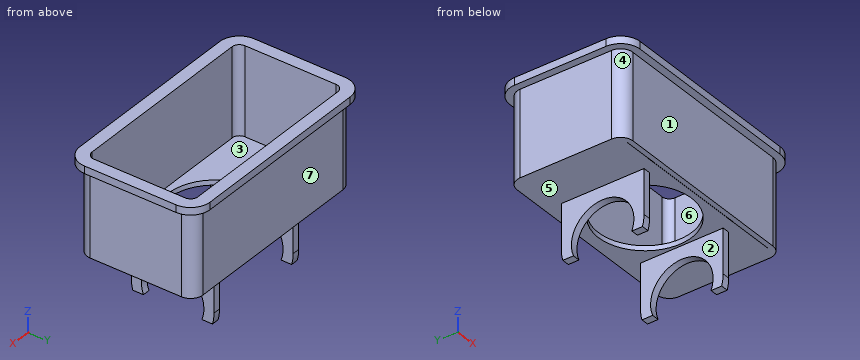
from build123d import *

# Parameters (mm, degrees)
BOSS_EXTRUDE1_DEPTH = 3
BOSS_EXTRUDE2_START = -38
BOSS_EXTRUDE2_DEPTH = 38
SKETCH3_R           = 19
BOSS_EXTRUDE3_DEPTH = 2
SKETCH4_W           = 3
SKETCH4_H           = 42
BOSS_EXTRUDE4_DEPTH = 35
CUT_EXTRUDE1_START  = -46
SKETCH5_R           = 12.75
CUT_EXTRUDE1_DEPTH  = 46
CUT_EXTRUDE2_REACH  = 103.826
CUT_EXTRUDE3_REACH  = 103.826
SKETCH7_W           = 14.582252834
SKETCH7_H           = 33.756


with BuildPart() as part:
    # Sketch1 → Boss-Extrude1 (new body)
    with BuildSketch(Plane.XY):
        with BuildLine():
            Line((-38, 26.6), (38, 26.6))
            ThreePointArc((38, 26.6), (43.656854249, 24.256854249), (46, 18.6))
            Line((46, 18.6), (46, -18.6))
            ThreePointArc((46, -18.6), (43.656854249, -24.256854249), (38, -26.6))
            Line((38, -26.6), (-38, -26.6))
            ThreePointArc((-38, -26.6), (-43.656854249, -24.256854249), (-46, -18.6))
            Line((-46, -18.6), (-46, 18.6))
            ThreePointArc((-46, 18.6), (-43.656854249, 24.256854249), (-38, 26.6))
        make_face()
        with BuildLine():
            Line((-38, -23.6), (38, -23.6))
            ThreePointArc((38, -23.6), (41.535533906, -22.135533906), (43, -18.6))
            Line((43, -18.6), (43, 18.6))
            ThreePointArc((43, 18.6), (41.535533906, 22.135533906), (38, 23.6))
            Line((38, 23.6), (-38, 23.6))
            ThreePointArc((-38, 23.6), (-41.535533906, 22.135533906), (-43, 18.6))
            Line((-43, 18.6), (-43, -18.6))
            ThreePointArc((-43, -18.6), (-41.535533906, -22.135533906), (-38, -23.6))
        make_face(mode=Mode.SUBTRACT)
    extrude(amount=BOSS_EXTRUDE1_DEPTH)

    # Sketch2 → Boss-Extrude2 (add)
    with BuildSketch(Plane.XY.offset(3).offset(BOSS_EXTRUDE2_START)):
        with BuildLine():
            Line((43, 18.6), (43, -18.6))
            ThreePointArc((43, -18.6), (41.535533906, -22.135533906), (38, -23.6))
            Line((38, -23.6), (-38, -23.6))
            ThreePointArc((-38, -23.6), (-41.535533906, -22.135533906), (-43, -18.6))
            Line((-43, -18.6), (-43, 18.6))
            ThreePointArc((-43, 18.6), (-41.535533906, 22.135533906), (-38, 23.6))
            Line((-38, 23.6), (38, 23.6))
            ThreePointArc((38, 23.6), (41.535533906, 22.135533906), (43, 18.6))
        make_face()
        with BuildLine():
            ThreePointArc((41, 18.6), (40.121320344, 20.721320344), (38, 21.6))
            Line((38, 21.6), (-38, 21.6))
            ThreePointArc((-38, 21.6), (-40.121320344, 20.721320344), (-41, 18.6))
            Line((-41, 18.6), (-41, -18.6))
            ThreePointArc((-41, -18.6), (-40.121320344, -20.721320344), (-38, -21.6))
            Line((-38, -21.6), (38, -21.6))
            ThreePointArc((38, -21.6), (40.121320344, -20.721320344), (41, -18.6))
            Line((41, -18.6), (41, 18.6))
        make_face(mode=Mode.SUBTRACT)
    extrude(amount=BOSS_EXTRUDE2_DEPTH)

    # Sketch3 → Boss-Extrude3 (add)
    with BuildSketch(Plane(origin=(0, 0, -35), x_dir=(-1, 0, 0), z_dir=(0, 0, -1))):
        with BuildLine():
            ThreePointArc((41, 18.6), (40.121320344, 20.721320344), (38, 21.6))
            Line((38, 21.6), (-38, 21.6))
            ThreePointArc((-38, 21.6), (-40.121320344, 20.721320344), (-41, 18.6))
            Line((-41, 18.6), (-41, -18.6))
            ThreePointArc((-41, -18.6), (-40.365961681, -20.444512219), (-38.731849783, -21.509363486))
            Line((-38.731849783, -21.509363486), (38.731849783, -21.509363486))
            ThreePointArc((38.731849783, -21.509363486), (40.365961681, -20.444512219), (41, -18.6))
            Line((41, -18.6), (41, 18.6))
        make_face()
        Circle(SKETCH3_R, mode=Mode.SUBTRACT)
    extrude(amount=-BOSS_EXTRUDE3_DEPTH)

    # Sketch4 → Boss-Extrude4 (add)
    with BuildSketch(Plane(origin=(0, 0, -35), x_dir=(-1, 0, 0), z_dir=(0, 0, -1))):
        with Locations((-21.5, 2.6)):
            Rectangle(SKETCH4_W, SKETCH4_H)
        with Locations((21.5, 2.6)):
            Rectangle(SKETCH4_W, SKETCH4_H)
    extrude(amount=BOSS_EXTRUDE4_DEPTH)

    # Sketch5 → Cut-Extrude1 (cut)
    with BuildSketch(Plane.ZY.offset(23).offset(CUT_EXTRUDE1_START)):
        with Locations(Location((-53.122, 0, 0), (0, 0, 270))):
            Circle(SKETCH5_R)
    extrude(amount=CUT_EXTRUDE1_DEPTH, mode=Mode.SUBTRACT)

    # Cut-Extrude2: up to this face of the body (flat: up to its plane)
    cut_extrude2_end = Plane(part.part.faces().sort_by_distance((23, -17.853282523, -52.5))[0])
    # Sketch6 → Cut-Extrude2 (cut, up to the picked face)
    with BuildSketch(Plane.ZY.offset(23), mode=Mode.PRIVATE) as cut_extrude2_sk1:
        with BuildLine():
            ThreePointArc((-53.122, -16.878), (-65.056548253, -11.934548253), (-70, 0))
            Line((-70, 0), (-70, -18.4))
            Line((-70, -18.4), (-35, -18.4))
            Line((-35, -18.4), (-35, -16.878))
            Line((-35, -16.878), (-53.122, -16.878))
        make_face()
    cut_extrude2_tool1 = split(extrude(cut_extrude2_sk1.sketch, amount=-CUT_EXTRUDE2_REACH, mode=Mode.PRIVATE), bisect_by=cut_extrude2_end, keep=Keep.BOTH, mode=Mode.PRIVATE)
    # Sketch6 → Cut-Extrude2 (cut, up to the picked face)
    with BuildSketch(Plane.ZY.offset(23), mode=Mode.PRIVATE) as cut_extrude2_sk2:
        with BuildLine():
            ThreePointArc((-70, 0), (-65.056548253, 11.934548253), (-53.122, 16.878))
            Line((-53.122, 16.878), (-35, 16.878))
            Line((-35, 16.878), (-35, 23.6))
            Line((-35, 23.6), (-70, 23.6))
            Line((-70, 23.6), (-70, 0))
        make_face()
    cut_extrude2_tool2 = split(extrude(cut_extrude2_sk2.sketch, amount=-CUT_EXTRUDE2_REACH, mode=Mode.PRIVATE), bisect_by=cut_extrude2_end, keep=Keep.BOTH, mode=Mode.PRIVATE)
    add(cut_extrude2_tool1.solids().sort_by(Axis((-23, -12.214152, -65.336152), (1, 0, 0)))[0], mode=Mode.SUBTRACT)
    add(cut_extrude2_tool2.solids().sort_by(Axis((-23, 18.768234, -55.331805), (1, 0, 0)))[0], mode=Mode.SUBTRACT)

    # Cut-Extrude3: up to this face of the body (flat: up to its plane)
    cut_extrude3_end = Plane(part.part.faces().sort_by_distance((23, 0, -35.486257909))[0])
    # Sketch7 → Cut-Extrude3 (cut, up to the picked face)
    with BuildSketch(Plane.ZY.offset(23), mode=Mode.PRIVATE) as cut_extrude3_sk1:
        with Locations((-64.958043362, 0)):
            Rectangle(SKETCH7_W, SKETCH7_H)
    cut_extrude3_tool1 = split(extrude(cut_extrude3_sk1.sketch, amount=-CUT_EXTRUDE3_REACH, mode=Mode.PRIVATE), bisect_by=cut_extrude3_end, keep=Keep.BOTH, mode=Mode.PRIVATE)
    add(cut_extrude3_tool1.solids().sort_by(Axis((-23, 0, -64.958043), (1, 0, 0)))[0], mode=Mode.SUBTRACT)


solid = part.part
Geometry check sheet. Reference: the model listing, model coordinates, mm. Face numbers are marked on the shaded views. A direction names the side the tool comes from. Give positions to 0.01 mm unless a question says otherwise; leave off trailing zeros. Loops run counter-clockwise (first coordinate to the right, second up) from the corner with the lowest first, then second, coordinate; pieces in that order, holes last. Notation, with made-up numbers: M 50,-18 L 83,-18 A16 ccw 83,-13 Z; hole C 36,68 d8. An arc over 180 degrees is marked long. Answer as a JSON object with one key per item and string values. Group by question number.
Item 1: Gauge pin test, flat ends, axial feed: pin 1 (4 mm diameter, centred on y = 0, z = -40, fed in from +X); pin 2 (3.5 mm diameter, centred on x = -21.5, z = -47, fed in from +Y); pin 3 (3 mm diameter, centred on x = 17.5, z = -48.5, fed in from -Y); pin 4 (4 mm diameter, centred on y = 15, z = -17.5, fed in from +X). Record the tip position at first contact, or that the pin passes through.
Item 2: Sectioned sample at A-A on z = -30.5. Record the boundary of the cut face in (x, y).
Item 3: Sectioned sample at D-D on z = -45.5. Record the boundary of the cut face in (x, y), plus the area to 3 significant figures.
Item 4: Sectioned sample at B-B on x = 0. Record the boundary of the cut face in (y, z), plus the area to 3 significant figures.
Item 5: Sectioned sample at C-C on y = 0. Record the boundary of the cut face in (x, z), plus the area to 3 significant figures.
Item 6: Material ranges on L1, parallel to Y at x = -35, z = -21; L2, parallel to X at y = -16, z = -46; L3, parallel to X at y = 2, z = -19, recorded low to high.
Item 7: Mould release check, pull along Y, two halves, no side actions. Record for the marked faces 4, 5, 6 and 7: pulls with the +Y half, pulls with the -Y half, needs draft (parallel to the pull), parting line crosses it, or undercut.
Item 8: Access from +Z, -Z, +X, -X, +Y, -Y to the whole of each face (thin tool, end or side, straight path). Record for the marked faces 1, 2 and 3.
Findings below:
{
 "1": {"pin 1": "x = 23", "pin 2": "y = 16.88", "pin 3": "through", "pin 4": "x = 43"},
 "2": {"outline": "M -43,-18.6 A5 ccw -38,-23.6 L 38,-23.6 A5 ccw 43,-18.6 L 43,18.6 A5 ccw 38,23.6 L -38,23.6 A5 ccw -43,18.6 Z; hole M -41,-18.6 A3 ccw -38,-21.6 L 38,-21.6 A3 ccw 41,-18.6 L 41,18.6 A3 ccw 38,21.6 L -38,21.6 A3 ccw -41,18.6 Z"},
 "3": {"outline": "M -23,-16.88 L -20,-16.88 L -20,-10.22 L -23,-10.22 Z; M -23,10.22 L -20,10.22 L -20,16.88 L -23,16.88 Z; M 20,-16.88 L 23,-16.88 L 23,-10.22 L 20,-10.22 Z; M 20,10.22 L 23,10.22 L 23,16.88 L 20,16.88 Z", "area": "79.9 mm2"},
 "4": {"outline": "M -26.6,0 L -23.6,0 L -23.6,-35 L -21.6,-35 L -21.6,3 L -26.6,3 Z; M -21.51,-35 L -19,-35 L -19,-33 L -21.51,-33 Z; M 19,-35 L 23.6,-35 L 23.6,0 L 26.6,0 L 26.6,3 L 21.6,3 L 21.6,-33 L 19,-33 Z", "area": "180 mm2"},
 "5": {"outline": "M -46,0 L -43,0 L -43,-35 L -23,-35 L -23,-40.37 L -20,-40.37 L -20,-35 L -19,-35 L -19,-33 L -41,-33 L -41,3 L -46,3 Z; M 19,-35 L 20,-35 L 20,-40.37 L 23,-40.37 L 23,-35 L 43,-35 L 43,0 L 46,0 L 46,3 L 41,3 L 41,-33 L 19,-33 Z", "area": "290 mm2"},
 "6": {"L1": "-23.6 to -21.6, 21.6 to 23.6", "L2": "-23 to -20, 20 to 23", "L3": "-43 to -41, 41 to 43"},
 "7": {"face 4": "pulls with the -Y half", "face 5": "needs draft", "face 6": "undercut", "face 7": "pulls with the +Y half"},
 "8": {"face 1": "-Z, +X, -X, -Y", "face 2": "-Z, +Y, -Y", "face 3": "+Z"}
}
